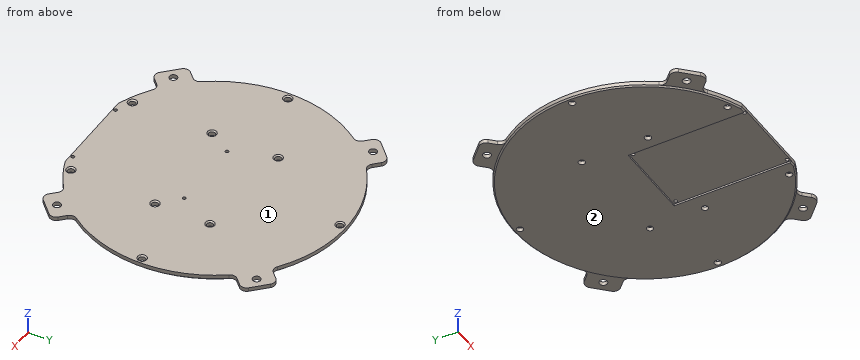
from build123d import *

# Parameters (mm, degrees)
ESBO_O1_R                = 2.5
ESBO_O1_W                = 61
ESBO_O1_H                = 90.5
ESBO_O1_R_2              = 1.3
RESSALTO_EXTRUS_O1_DEPTH = 4
ESBO_O1_4_W              = 61
ESBO_O1_4_H              = 90.5
ESBO_O1_4_R              = 1.3
CORTE_EXTRUS_O3_DEPTH    = 1.5
RESSALTO_EXTRUS_O3_START = -3
ESBO_O2_R                = 3
RESSALTO_EXTRUS_O3_DEPTH = 3
CHANFRO1_SIZE            = 1
CHANFRO2_SIZE            = 1


with BuildPart() as part:
    # Esboço1 → Ressalto-extrusão1 (new body)
    # profile 1 of 2: a face of its own
    with BuildSketch(Plane.XY):
        with BuildLine():
            Line((-35.106979363, -95.235235076), (-30.5, -95.235235076))
            Line((-30.5, -95.235235076), (-30.5, -4.735235076))
            Line((-30.5, -4.735235076), (30.5, -4.735235076))
            Line((30.5, -4.735235076), (30.5, -95.235235076))
            Line((30.5, -95.235235076), (35.106979363, -95.235235076))
            ThreePointArc((35.106979363, -95.235235076), (0, 101.5), (-35.106979363, -95.235235076))
        make_face()
        with Locations((-40.782662258, -87.458701449)):
            Circle(ESBO_O1_R, mode=Mode.SUBTRACT)
        with Locations((-96.5, 0)):
            Circle(ESBO_O1_R, mode=Mode.SUBTRACT)
        with Locations((-39.78606917, -25.45794308)):
            Circle(ESBO_O1_R, mode=Mode.SUBTRACT)
        with Locations((40.782662258, -87.458701449)):
            Circle(ESBO_O1_R, mode=Mode.SUBTRACT)
        with Locations((42.90493083, -21.30794308)):
            Circle(ESBO_O1_R, mode=Mode.SUBTRACT)
        with Locations((96.5, 0)):
            Circle(ESBO_O1_R, mode=Mode.SUBTRACT)
        with Locations((-39.78606917, 25.605133502)):
            Circle(ESBO_O1_R, mode=Mode.SUBTRACT)
        with Locations((42.90493083, 21.118210084)):
            Circle(ESBO_O1_R, mode=Mode.SUBTRACT)
        with Locations((0, 96.5)):
            Circle(ESBO_O1_R, mode=Mode.SUBTRACT)
    # profile 2 of 2: a face of its own
    with BuildSketch(Plane.XY):
        with Locations((0, -49.985235076)):
            Rectangle(ESBO_O1_W, ESBO_O1_H)
        with Locations((-28.25, -93.235235076)):
            Circle(ESBO_O1_R_2, mode=Mode.SUBTRACT)
        with Locations((-28.25, -7.235235076)):
            Circle(ESBO_O1_R_2, mode=Mode.SUBTRACT)
        with Locations((28.25, -93.235235076)):
            Circle(ESBO_O1_R_2, mode=Mode.SUBTRACT)
        with Locations((28.25, -7.235235076)):
            Circle(ESBO_O1_R_2, mode=Mode.SUBTRACT)
    extrude(amount=RESSALTO_EXTRUS_O1_DEPTH)

    # Esboço1<4> → Corte-extrusão3 (cut)
    with BuildSketch(Plane.XY):
        with Locations((0, -49.985235076)):
            Rectangle(ESBO_O1_4_W, ESBO_O1_4_H)
        with Locations((-28.25, -93.235235076)):
            Circle(ESBO_O1_4_R, mode=Mode.SUBTRACT)
        with Locations((-28.25, -7.235235076)):
            Circle(ESBO_O1_4_R, mode=Mode.SUBTRACT)
        with Locations((28.25, -93.235235076)):
            Circle(ESBO_O1_4_R, mode=Mode.SUBTRACT)
        with Locations((28.25, -7.235235076)):
            Circle(ESBO_O1_4_R, mode=Mode.SUBTRACT)
    extrude(amount=CORTE_EXTRUS_O3_DEPTH, mode=Mode.SUBTRACT)

    # Esboço2 → Ressalto-extrusão3 (add)
    # profile 1 of 4: a face of its own
    with BuildSketch(Plane.XY.offset(4).offset(RESSALTO_EXTRUS_O3_START)):
        with BuildLine():
            ThreePointArc((-59.002353185, -82.589177975), (-71.77133829, -71.77133829), (-82.589177975, -59.002353185))
            ThreePointArc((-82.589177975, -59.002353185), (-81.674630343, -62.321074298), (-83.122076482, -65.444406952))
            Line((-83.122076482, -65.444406952), (-87.681240867, -70.003571337))
            ThreePointArc((-87.681240867, -70.003571337), (-89.145706961, -73.539105243), (-87.681240867, -77.074639149))
            Line((-87.681240867, -77.074639149), (-82.377940008, -82.377940008))
            Line((-82.377940008, -82.377940008), (-77.074639149, -87.681240867))
            ThreePointArc((-77.074639149, -87.681240867), (-73.539105243, -89.145706961), (-70.003571337, -87.681240867))
            Line((-70.003571337, -87.681240867), (-65.444406952, -83.122076482))
            ThreePointArc((-65.444406952, -83.122076482), (-62.321074298, -81.674630343), (-59.002353185, -82.589177975))
        make_face()
        with Locations((-77.074639149, -77.074639149)):
            Circle(ESBO_O2_R, mode=Mode.SUBTRACT)
    # profile 2 of 4: a face of its own
    with BuildSketch(Plane.XY.offset(4).offset(RESSALTO_EXTRUS_O3_START)):
        with BuildLine():
            ThreePointArc((-82.589177975, 59.002353185), (-71.77133829, 71.77133829), (-59.002353185, 82.589177975))
            ThreePointArc((-59.002353185, 82.589177975), (-62.321074298, 81.674630343), (-65.444406952, 83.122076482))
            Line((-65.444406952, 83.122076482), (-70.003571337, 87.681240867))
            ThreePointArc((-70.003571337, 87.681240867), (-73.539105243, 89.145706961), (-77.074639149, 87.681240867))
            Line((-77.074639149, 87.681240867), (-82.377940008, 82.377940008))
            Line((-82.377940008, 82.377940008), (-87.681240867, 77.074639149))
            ThreePointArc((-87.681240867, 77.074639149), (-89.145706961, 73.539105243), (-87.681240867, 70.003571337))
            Line((-87.681240867, 70.003571337), (-83.122076482, 65.444406952))
            ThreePointArc((-83.122076482, 65.444406952), (-81.674630343, 62.321074298), (-82.589177975, 59.002353185))
        make_face()
        with Locations((-77.074639149, 77.074639149)):
            Circle(ESBO_O2_R, mode=Mode.SUBTRACT)
    # profile 3 of 4: a face of its own
    with BuildSketch(Plane.XY.offset(4).offset(RESSALTO_EXTRUS_O3_START)):
        with BuildLine():
            ThreePointArc((59.002353185, 82.589177975), (71.77133829, 71.77133829), (82.589177975, 59.002353185))
            ThreePointArc((82.589177975, 59.002353185), (81.674630343, 62.321074298), (83.122076482, 65.444406952))
            Line((83.122076482, 65.444406952), (87.681240867, 70.003571337))
            ThreePointArc((87.681240867, 70.003571337), (89.145706961, 73.539105243), (87.681240867, 77.074639149))
            Line((87.681240867, 77.074639149), (82.377940008, 82.377940008))
            Line((82.377940008, 82.377940008), (77.074639149, 87.681240867))
            ThreePointArc((77.074639149, 87.681240867), (73.539105243, 89.145706961), (70.003571337, 87.681240867))
            Line((70.003571337, 87.681240867), (65.444406952, 83.122076482))
            ThreePointArc((65.444406952, 83.122076482), (62.321074298, 81.674630343), (59.002353185, 82.589177975))
        make_face()
        with Locations((77.074639149, 77.074639149)):
            Circle(ESBO_O2_R, mode=Mode.SUBTRACT)
    # profile 4 of 4: a face of its own
    with BuildSketch(Plane.XY.offset(4).offset(RESSALTO_EXTRUS_O3_START)):
        with BuildLine():
            Line((77.074639149, -87.681240867), (82.377940008, -82.377940008))
            Line((82.377940008, -82.377940008), (87.681240867, -77.074639149))
            ThreePointArc((87.681240867, -77.074639149), (89.145706961, -73.539105243), (87.681240867, -70.003571337))
            Line((87.681240867, -70.003571337), (83.122076482, -65.444406952))
            ThreePointArc((83.122076482, -65.444406952), (81.674630343, -62.321074298), (82.589177975, -59.002353185))
            ThreePointArc((82.589177975, -59.002353185), (71.77133829, -71.77133829), (59.002353185, -82.589177975))
            ThreePointArc((59.002353185, -82.589177975), (62.321074298, -81.674630343), (65.444406952, -83.122076482))
            Line((65.444406952, -83.122076482), (70.003571337, -87.681240867))
            ThreePointArc((70.003571337, -87.681240867), (73.539105243, -89.145706961), (77.074639149, -87.681240867))
        make_face()
        with Locations((77.074639149, -77.074639149)):
            Circle(ESBO_O2_R, mode=Mode.SUBTRACT)
    extrude(amount=RESSALTO_EXTRUS_O3_DEPTH)

    # Chanfro1
    chanfro1_edges = [part.edges().sort_by_distance(p)[0] for p in [
        (-32.803489682, -95.235235076, 0),
        (0, 101.5, 0),
        (32.803489682, -95.235235076, 0),
    ]]
    chamfer(chanfro1_edges, length=CHANFRO1_SIZE - 0.0001)  # a hair under: the kernel refuses the full size

    # Chanfro2
    chanfro2_edges = [part.edges().sort_by_distance(p)[0] for p in [
        (38.282662258, -87.458701449, 4),
        (40.40493083, -21.30794308, 4),
        (94, 0, 4),
        (40.40493083, 21.118210084, 4),
        (-2.5, 96.5, 4),
        (-42.28606917, 25.605133502, 4),
        (-42.28606917, -25.45794308, 4),
        (-99, 0, 4),
        (-43.282662258, -87.458701449, 4),
    ]]
    chamfer(chanfro2_edges, length=CHANFRO2_SIZE)


solid = part.part
CAD build for the part. Positions are in the model's coordinates, mm. Face numbers are marked on the shaded views. Round coordinates to 2 decimals unless told otherwise and drop trailing zeros. Order: outer loops, then holes, each group sorted by start corner. A loop starts at its lowest first (then second) coordinate and runs counter-clockwise, first axis right, second up. Notation, with made-up numbers: (75.25, 9.5) -> (122.25, 9.5) arc R16 cw to (122.25, 38.5) -> close; hole circle Ø4 at (-10.75, -15.5). An arc over 180 degrees is marked (long way). Write item = value, one per line. Start each with the question number.
(1) Pull direction Z, two halves, no side cores. Call the marked faces 1 and 2: released by +Z, released by -Z, zero draft, split by the parting line, or undercut.
(2) Probe line 1 (Y direction, x = -40, z = 3.4); line 2 (Y direction, x = -28.25, z = 2.35); line 3 (Y direction, x = 78.5, z = 3.3). List the from-to ranges inside material, lowest first. Write a range as [from, to].
(3) Pin check, flat tips, straight feed: P1, Ø4, axis at x = 0, y = 96.5, coming from the -Z side; P2, Ø1.5, axis at x = 17.5, y = -29, coming from the -Z side; P3, Ø1.2, axis at y = -43.5, z = 1, coming from the +X side; P4, Ø7, axis at x = 77.07, y = 77.07, coming from the -Z side. Stop position of each tip, or through.
(4) Cut at B-B, the plane x = 0. List the corners of the cut face in (y, z).
(5) Cut at A-A, the plane y = 0. List the corners of the cut face in (x, z).
Model answer:
q1.face_1 = released by +Z
q1.face_2 = released by -Z
q2.line_1 = [-93.29, -90.25], [-84.67, -28.35], [-22.57, 22.71], [28.5, 93.29]
q2.line_2 = [-95.24, -94.54], [-91.94, -8.54], [-5.94, 97.49]
q2.line_3 = [-86.26, -79.71], [-74.43, 74.43], [79.71, 86.26]
q3.P1 = through
q3.P2 = 1.5
q3.P3 = 91.99
q3.P4 = 1
q4.outline = (-95.24, 1.5) -> (-4.74, 1.5) -> (-4.74, 0) -> (94, 0) -> (94, 3) -> (93, 4) -> (-95.24, 4) -> close; (99, 0) -> (100.5, 0) -> (101.5, 1) -> (101.5, 4) -> (100, 4) -> (99, 3) -> close
q5.outline = (-101.5, 1) -> (-100.5, 0) -> (-99, 0) -> (-99, 3) -> (-100, 4) -> (-101.5, 4) -> close; (-94, 0) -> (94, 0) -> (94, 3) -> (93, 4) -> (-93, 4) -> (-94, 3) -> close; (99, 0) -> (100.5, 0) -> (101.5, 1) -> (101.5, 4) -> (100, 4) -> (99, 3) -> close
